```python
from build123d import *

# Parameters (mm, degrees)
VYSUNOUT1_DEPTH          = 8
ZAOBLIT1_R               = 5
ZAOBLIT2_R               = 3
SKICA2_W                 = 11
SKICA2_H                 = 22
ODEBRAT_VYSUNUT_M1_DEPTH = 12
ZAOBLIT3_R               = 3.5


with BuildPart() as part:
    # Skica1 → Vysunout1 (new body, symmetric)
    with BuildSketch(Plane(origin=(0, 0, 0), x_dir=(0, 0, -1), z_dir=(1, 0, 0))):
        with BuildLine():
            Line((-20.1, 0), (-20.1, 22))
            Line((-20.1, 22), (-15.1, 22))
            Line((-15.1, 22), (-15.1, 7.630965))
            ThreePointArc((-15.1, 7.630965), (-7.868346, 4.330613), (0, 3.2))
            ThreePointArc((0, 3.2), (7.868346, 4.330613), (15.1, 7.630965))
            Line((15.1, 7.630965), (15.1, 22))
            Line((15.1, 22), (20.1, 22))
            Line((20.1, 22), (20.1, 9))
            Line((20.1, 9), (23.564102, 3))
            ThreePointArc((23.564102, 3), (22.802361, -1.949109), (17.805694, -2.276608))
            Line((17.805694, -2.276608), (14.144179, 0.287213))
            ThreePointArc((14.144179, 0.287213), (7.238589, -2.019217), (0, -2.8))
            ThreePointArc((0, -2.8), (-6.893657, -2.09263), (-13.5, 0))
            Line((-13.5, 0), (-20.1, 0))
        make_face()
    extrude(amount=VYSUNOUT1_DEPTH, both=True)

    # Zaoblit1
    zaoblit1_edges = [part.edges().sort_by_distance(p)[0] for p in [
        (-8, 22, 17.6),
        (-8, 22, -17.6),
        (8, 22, -17.6),
        (8, 22, 17.6),
    ]]
    fillet(zaoblit1_edges, radius=ZAOBLIT1_R)

    # Zaoblit2
    zaoblit2_edges = [part.edges().sort_by_distance(p)[0] for p in [
        (-4, 0, 20.1),
    ]]
    fillet(zaoblit2_edges, radius=ZAOBLIT2_R)

    # Skica2 → Odebrat vysunutím1 (cut, through all)
    with BuildSketch(Plane(origin=(0, 8, 0), x_dir=(-1, 0, 0), z_dir=(0, 1, 0))):
        Rectangle(SKICA2_W, SKICA2_H)
    extrude(amount=-ODEBRAT_VYSUNUT_M1_DEPTH, mode=Mode.SUBTRACT)

    # Zaoblit3
    zaoblit3_edges = [part.edges().sort_by_distance(p)[0] for p in [
        (-5.5, 2.2439, -11),
        (5.5, 2.2439, -11),
        (5.5, 2.2439, 11),
        (-5.5, 2.2439, 11),
    ]]
    fillet(zaoblit3_edges, radius=ZAOBLIT3_R)


solid = part.part
```
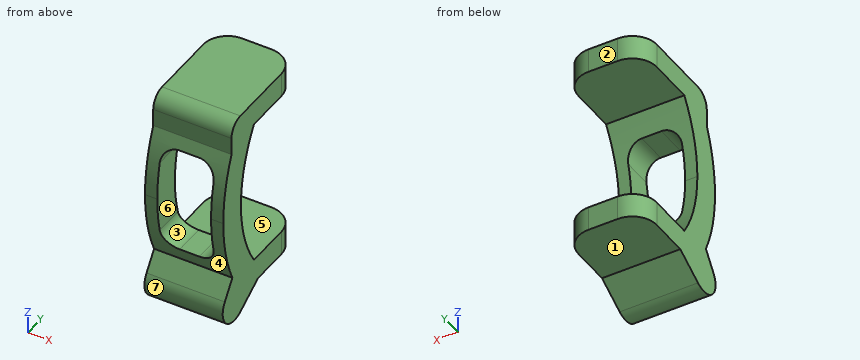
Source: CAD feature listing. Evaluate the final solid. Frame: model axes, mm. Face numbers are marked on the shaded views. A direction names the side the tool comes from. Give positions to 0.01 mm unless a question says otherwise; leave off trailing zeros. Order: outer loops, then holes, each group sorted by start corner. A loop starts at its lowest first (then second) coordinate and runs counter-clockwise, first axis right, second up.
(1) Section query C-C (z = -2). Return the cut outline in (x, y), plus the area to 3 significant figures.
(2) Section query B-B (x = 1). Return the cut outline in (y, z).
(3) Pull-direction query (Z, two-part tool) for the marked faces 1, 2 and 3; classes: +Z half, -Z half, draft (parallel to the pull), parting line (faces both ways), or undercut.
(4) Section query D-D (x = 6). Return the cut outline in (y, z), plus the area to 3 significant figures.
(5) Section query A-A (y = 14). Return the cut outline in (x, z).
(6) Material intervals for line 1 along Z through (x, y) = (1.75, 13); line 2 along Y through (x, z) = (-1.25, 16); line 3 along Y through (x, z) = (2, -11.5), sorted ascending.
(7) Access query for the marked faces 4, 5, 6 and 7. Directions: +Z, -Z, +X, -X, +Y, -Y. A direction counts if a zero-diameter tool reaches every point of the face in a straight line with its end or side. Return the directions, or none.
(8) Contact query for flat-ended pins moving along their axis: P1, Ø6, axis at x = -5, z = 7.5, coming from the +Y side; P2, Ø4, axis at x = 3, z = 15, coming from the -Y side; P3, Ø4.5, axis at x = 0.5, y = 3.5, coming from the -Z side. Output: stop coordinate, or through.
Outcome:
1. outline: (-8, -2.74) - (-5.5, -2.74) - (-5.5, 3.27) - (-8, 3.27) - close; (5.5, -2.74) - (8, -2.74) - (8, 3.27) - (5.5, 3.27) - close
1. area: 30.1 mm2
2. outline: (-2.28, -17.81) arc R4 ccw to (3, -23.56) - (9, -20.1) - (22, -20.1) - (22, -15.1) - (7.63, -15.1) arc R27.94 cw to (5.46, -11) - (-0.97, -11) arc R33.94 ccw to (0.29, -14.14) - close; (-0.97, 11) - (5.46, 11) arc R27.94 cw to (7.63, 15.1) - (22, 15.1) - (22, 20.1) - (3, 20.1) arc R3 ccw to (0, 17.1) - (0, 13.5) arc R33.94 ccw to start
3. face 1: -Z half
3. face 2: draft
3. face 3: undercut
4. outline: (-2.8, 0) arc R33.94 ccw to (0.29, -14.14) - (-2.28, -17.81) arc R4 ccw to (3, -23.56) - (9, -20.1) - (21, -20.1) - (21, -15.1) - (7.63, -15.1) arc R27.94 cw to (3.2, 0) arc R27.94 cw to (7.63, 15.1) - (21, 15.1) - (21, 20.1) - (3, 20.1) arc R3 ccw to (0, 17.1) - (0, 13.5) arc R33.94 ccw to start
4. area: 439 mm2
5. outline: (-8, -20.1) - (8, -20.1) - (8, -15.1) - (-8, -15.1) - close; (-8, 15.1) - (8, 15.1) - (8, 20.1) - (-8, 20.1) - close
6. line 1: z = -20.1 to -15.1, 15.1 to 20.1
6. line 2: y = 0 to 22
6. line 3: y = -0.79 to 5.68
7. face 4: +X, -X, -Y
7. face 5: +X, -X, +Y
7. face 6: +Y, -Y
7. face 7: +X, -X
8. P1: stops at y = 5.25
8. P2: stops at y = -0.21
8. P3: stops at z = -24.09
